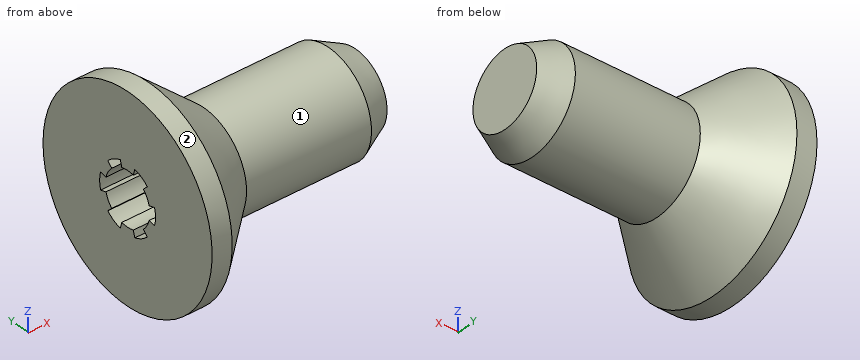
Autodesk Inventor part; units mm, degrees
ref_plane "Work Plane1" through (66.6877, 0, 0) normal (0, 0, -1) x (1, 0, 0)
ref_plane "YZ Plane" through (0, 0, 0) normal (1, 0, 0) x (0, 1, 0)
ref_plane "XZ Plane" through (0, 0, 0) normal (0, 1, 0) x (-1, 0, 0)
sketch "Szkic1" plane through (0, 0, 0) normal (0, 0, 1) x (1, 0, 0)
  line L0 (6.35, 0) -> (6.35, 1.4224)
  line L1 (6.35, 1.4224) -> (2.1082, 1.4224)
  line L2 (0, 2.7686) -> (0, 0.9144)
  line L3 (0, 0.9144) -> (1.397, 0.9144)
  line L4 (1.397, 0.9144) -> (1.9249, 0)
  line L5 (1.9249, 0) -> (6.35, 0)
  line L6 (0, 2.7686) -> (0.5596, 2.7686)
  line L7 (0.5596, 2.7686) -> (2.1082, 1.4224)
  line L8 (-1.27, 0) -> (7.62, 0)
  line L9 (0, -0.5537) -> (0, 3.3223)
  dimension "d0" = 6.35
  dimension "d1" = 1.397
  dimension "d2" = 2.8448
  dimension "d3" = 2.1082
  dimension "d4" = 41
  dimension "d5" = 1.8288
  dimension "d6" = 60
  dimension "d7" = 5.5372
revolve "Bryła" add sketch "Szkic1" angle 360 about axis through (1.9249, 0, 0) along (1, 0, 0) contours L5 L4 L3 L2 L6 L7 L1 L0
sketch "Szkic2" plane through (0, 0, 0) normal (-1, 0, 0) x (0, 0, 1)
  circle A0 centre (0, 0) radius 2.7686
  circle A1 centre (0, 0) radius 0.9144
  line L0 (0.7066, 0.1893) -> (0.8832, 0.2367)
  line L1 (0.7066, -0.1893) -> (0.8832, -0.2367)
  arc A2 (0.7066, -0.1893) -> (0.7066, 0.1893) centre (0, 0) ccw
  arc A3 (0.8832, -0.2367) -> (0.8832, 0.2367) centre (0, 0) ccw
  line L2 (0, -3.876) -> (0, 3.876)
  line L3 (-3.876, 0) -> (3.876, 0)
  line L4 (0.7066, 0.1893) -> (0, 0) construction
  line L5 (0, 0) -> (0.7066, -0.1893) construction
  line L6 (0.1893, 0.7066) -> (0.2367, 0.8832)
  line L7 (0.5173, 0.5173) -> (0.6466, 0.6466)
  arc A4 (0.5173, 0.5173) -> (0.1893, 0.7066) centre (0, 0) ccw
  arc A5 (0.6466, 0.6466) -> (0.2367, 0.8832) centre (0, 0) ccw
  line L8 (-0.5173, 0.5173) -> (-0.6466, 0.6466)
  line L9 (-0.1893, 0.7066) -> (-0.2367, 0.8832)
  arc A6 (-0.1893, 0.7066) -> (-0.5173, 0.5173) centre (0, 0) ccw
  arc A7 (-0.2367, 0.8832) -> (-0.6466, 0.6466) centre (0, 0) ccw
  line L10 (-0.7066, -0.1893) -> (-0.8832, -0.2367)
  line L11 (-0.7066, 0.1893) -> (-0.8832, 0.2367)
  arc A8 (-0.7066, 0.1893) -> (-0.7066, -0.1893) centre (0, 0) ccw
  arc A9 (-0.8832, 0.2367) -> (-0.8832, -0.2367) centre (0, 0) ccw
  line L12 (-0.1893, -0.7066) -> (-0.2367, -0.8832)
  line L13 (-0.5173, -0.5173) -> (-0.6466, -0.6466)
  arc A10 (-0.5173, -0.5173) -> (-0.1893, -0.7066) centre (0, 0) ccw
  arc A11 (-0.6466, -0.6466) -> (-0.2367, -0.8832) centre (0, 0) ccw
  line L14 (0.5173, -0.5173) -> (0.6466, -0.6466)
  line L15 (0.1893, -0.7066) -> (0.2367, -0.8832)
  arc A12 (0.1893, -0.7066) -> (0.5173, -0.5173) centre (0, 0) ccw
  arc A13 (0.2367, -0.8832) -> (0.6466, -0.6466) centre (0, 0) ccw
  dimension "d8" = 1.463
  dimension "d9" = 1.8288
  dimension "d10" = 15
  dimension "d11" = 15
  dimension "d22" = 360
extrude "Szczelina" add sketch "Szkic2" against normal up to next contours L3 A2 L0 A1 | A1 L1 A2 L3 | L3 A8 L10 A1 | A1 L11 A8 L3 | A1 L7 A4 L6 | L9 A6 L8 A1 | A1 L13 A10 L12 | L15 A12 L14 A1
thread "Gwint"
chamfer "Faza1" distance 0.3785 distance2 0.7569 1 edges at (6.35, -1.4224, 0) measured on face at (6.35, -0.1427, 0.3949)
ref_plane "Work Plane1" through (66.6877, 0, 0) normal (0, 0, -1) x (1, 0, 0)
equation "\"d0\" = NLG"
equation "\"d1\" = INTI"
equation "\"d2\" = GD"
equation "\"d3\" = KOH"
equation "\"d4\" = 0.5 * SEWI"
equation "\"d5\" = SW"
equation "\"d7\" = KOD"
equation "\"d8\" = 0.8 * SW"
equation "\"d9\" = SW"
equation "\"d15\" = GEL"
equation "\"d17\" = -0.5 * SPD + 0.5 * GD"
equation "\"d18\" = GUL"
equation "\"NLG\" = 6.35"
equation "\"SW\" = 1.8288"
equation "\"INTI\" = 1.397"
equation "\"GEL\" = 2.6543"
equation "\"KOH\" = 2.1082"
equation "\"KOD\" = 5.5372"
equation "\"GUL\" = 0.75692"
equation "\"SPD\" = 2.08788"
equation "\"GD\" = NND"
equation "\"SEWI\" = 82deg"
equation "\"TOA\" = 30deg"
equation "\"GD1\" = SPD"
equation "\"EPV\" = 3.74448"
equation "\"THREADDIA\" = 2.8448"
equation "\"BDM\" = NND"
equation "\"NND\" = 2.8448"
equation "\"GAL\" = 1.5875"
equation "\"E0\" = 1.155 * SW"
properties part number "ANSI B18.3 - 4-40 UNC x 0,25" material "Stal, miękka"
CAD build for the part. Positions are in the model's coordinates, mm. Face numbers are marked on the shaded views. A direction names the side the tool comes from. Coordinates: 2 decimals unless noted, no trailing zeros. Order: outer loops, then holes, each group sorted by start corner. A loop starts at its lowest first (then second) coordinate and runs counter-clockwise, first axis right, second up. Notation, with made-up numbers: (16, 14.25) - (43, 14.25) arc R18 ccw to (43, 21.25) - close; hole circle Ø11 at (-26, 10). An arc over 180 degrees is marked (long way). Answer in a Markdown table with one row per item.
1. 3-axis set-ups, long thin cutter, end or side, ignore diameter. For the marked faces 1 and 2: which of +Z, -Z, +X, -X, +Y, -Y reach the whole face in a straight line?
Answer:
| item | result |
|---|---|
| face 1 | +X |
| face 2 | +X, -X |
2. Slice it at A-A, the plane x = 4.5. List the corners of the cut face in (y, z).
Answer:
| item | result |
|---|---|
| outline | circle Ø2.84 at (0, 0) |
3. Drill centre lines: L1, parallel to Z at x = 1.25, y = -0.05; L2, parallel to X at y = 0.5, z = 2.2; L3, parallel to Z at x = 2, y = 0.85. Where is each one in solid material? Low to high. Write a range as from..to.
Answer:
| item | result |
|---|---|
| L1 | -2.17..-0.73, 0.73..2.17 |
| L2 | 0..1.15 |
| L3 | -1.26..1.26 |
4. Flat gauge pins, fed straight in: P1, Ø1, axis at x = 5, z = -2, coming from the +Y side; P2, Ø3, axis at x = 5.5, y = -0.5, coming from the +Z side; P3, Ø2, axis at y = -2, z = 0.5, coming from the -X side. Where does each tip first touch, or does it go through?
Answer:
| item | result |
|---|---|
| P1 | through |
| P2 | z = 1.42 |
| P3 | x = 0 |
